from build123d import *

# Parameters (mm, degrees)
SKETCH1_W           = 120
SKETCH1_H           = 120
SKETCH1_R           = 25
BOSS_EXTRUDE1_DEPTH = 8
SKETCH2_R           = 1.65
CUT_EXTRUDE2_DEPTH  = 86.229103011
CIRPATTERN1_COUNT   = 6


with BuildPart() as part:
    # Sketch1 → Boss-Extrude1 (new body)
    with BuildSketch(Plane.XY):
        Rectangle(SKETCH1_W, SKETCH1_H)
        Circle(SKETCH1_R, mode=Mode.SUBTRACT)
    extrude(amount=BOSS_EXTRUDE1_DEPTH)

    # Sketch2 → Cut-Extrude2 (cut, through all)
    with BuildSketch(Plane.XY):
        with Locations((0, 32.5)):
            Circle(SKETCH2_R)
    cut_extrude2 = extrude(amount=CUT_EXTRUDE2_DEPTH, mode=Mode.SUBTRACT)

    # CirPattern1: Cut-Extrude2 ×6 about axis
    cirpattern1_axis = Axis((0, 0, 0), (0, 0, 1))
    for i in range(1, CIRPATTERN1_COUNT):
        add(cut_extrude2.rotate(cirpattern1_axis, i * 360 / CIRPATTERN1_COUNT), mode=Mode.SUBTRACT)


solid = part.part
Verification items for the finished model (mm, model axes). Give positions to 0.01 mm unless a question says otherwise; leave off trailing zeros. Loops run counter-clockwise (first coordinate to the right, second up) from the corner with the lowest first, then second, coordinate; pieces in that order, holes last.
1) Draft check along X on faces 1 (the cylindrical face through (29.72, -15.75, 3.94)), 2 (the flat face through (-28, 1, 0)), 3 (the flat face through (60, -1, 4)). Enter one of: pulls with the +X half, pulls with the -X half, needs draft (parallel to the pull), parting line crosses it, or undercut.
2) Thickness scan on line 1 along Y through (x, z) = (0, 5.75); line 2 along X through (y, z) = (32.5, 3); line 3 along X through (y, z) = (-12.5, 2). Record the ranges inside material, lowest first.
3) Sectioned sample at A-A, the plane x = 0. Enter the section's corners in (y, z).
4) Sectioned sample at D-D, the plane x = -21.5. Enter the section's corners in (y, z).
5) Depth check by flat-ended pin: pin 1 Ø3 at (x, y) = (0, -32.5) entering from +Z. Enter the tip coordinate at first touch or a pass-through.
6) Sectioned sample at C-C, the plane z = 1.75. Enter the section's corners in (x, y).
7) Sectioned sample at B-B, the plane y = 0. Enter the section's corners in (x, z).
Answers:
1. face 1: undercut
1. face 2: needs draft
1. face 3: pulls with the +X half
2. line 1: y = -60 to -34.15, -30.85 to -25, 25 to 30.85, 34.15 to 60
2. line 2: x = -60 to -1.65, 1.65 to 60
2. line 3: x = -60 to -21.65, 21.65 to 60
3. outline: (-60, 0) - (-34.15, 0) - (-34.15, 8) - (-60, 8) - close; (-30.85, 0) - (-25, 0) - (-25, 8) - (-30.85, 8) - close; (25, 0) - (30.85, 0) - (30.85, 8) - (25, 8) - close; (34.15, 0) - (60, 0) - (60, 8) - (34.15, 8) - close
4. outline: (-60, 0) - (-12.76, 0) - (-12.76, 8) - (-60, 8) - close; (12.76, 0) - (60, 0) - (60, 8) - (12.76, 8) - close
5. pin 1: passes through
6. outline: (-60, -60) - (60, -60) - (60, 60) - (-60, 60) - close; hole circle Ø3.3 at (-28.15, -16.25); hole circle Ø3.3 at (-28.15, 16.25); hole circle Ø50 at (0, 0); hole circle Ø3.3 at (0, -32.5); hole circle Ø3.3 at (0, 32.5); hole circle Ø3.3 at (28.15, -16.25); hole circle Ø3.3 at (28.15, 16.25)
7. outline: (-60, 0) - (-25, 0) - (-25, 8) - (-60, 8) - close; (25, 0) - (60, 0) - (60, 8) - (25, 8) - close
